Build history of the part. All positions in model axes, mm. A direction names the side the tool comes from. Give positions to 0.01 mm unless a question says otherwise; leave off trailing zeros. Loops run counter-clockwise (first coordinate to the right, second up) from the corner with the lowest first, then second, coordinate; pieces in that order, holes last. Notation, with made-up numbers: (35.25, -35.75) - (86.25, -35.75) arc R34 ccw to (86.25, -0.75) - close; hole circle Ø11 at (72, -7.75). An arc over 180 degrees is marked (long way). Return JSON: item names as keys, results as strings. Group by question number.
1) Drop flat-ended pins along their axis: pin 1 (3 mm diameter, centred on x = -4, z = 44, fed in from +Y); pin 2 (3 mm diameter, centred on x = -0.5, y = 0, fed in from +Z); pin 3 (6 mm diameter, centred on x = 3.5, z = 26, fed in from +Y). Give the stop position or say it passes through.
2) Mould opens along X. For faces 1 (the face through (0, -3, 75)), 2 (the face through (-5, 0, 37)), 3 (the face through (-0.151, 0.678, 16.986)) say: released by +X, released by -X, zero draft, split by the parting line, or undercut.
3) Drill centre lines: probe 1 along Y at (x, z) = (0, 3.5); probe 2 along Y at (x, z) = (-2, 69.5); probe 3 along Y at (x, z) = (-0.25, 28). Where is each one in solid material? Low to high. Write a range as from..to.
4) Slice it at A-A (z = 69.5). List the corners of the cut face in (x, y).
5) 3-axis set-ups, long thin cutter, end or side, ignore diameter. For faces 4 (the face through (0, 3, 75)), 5 (the face through (0, -2, 60)), 6 (the face through (0.867, 3.905, 7.605)): which of +Z, -Z, +X, -X, +Y, -Y reach the whole face in a straight line?
```python
from build123d import *

# Parameters (mm, degrees)
F0_R     = 5
F1_DEPTH = 75
F3_D     = 8
F3_DEPTH = 15
F3_TIP   = 2.4034424761
F4_W     = 2
F4_H     = 30
F5_DEPTH = 12.5


with BuildPart() as f1:
    # F0 (on Top) → F1 (new body)
    with BuildSketch(Plane.XY):
        Circle(F0_R)
    extrude(amount=F1_DEPTH)

    # F3
    with Locations(Plane(origin=(0, 0, 0), x_dir=(1, 0, 0), z_dir=(0, 0, -1))):
        with Locations((0, 0)):
            Hole(F3_D / 2, depth=F3_DEPTH)
            with Locations((0, 0, -(F3_DEPTH + F3_TIP / 2))):  # 118° drill point
                Cone(0, F3_D / 2, F3_TIP, mode=Mode.SUBTRACT)

    # F4 (on Right) → F5 (cut, symmetric)
    with BuildSketch(Plane.YZ):
        with Locations((-1, 60)):
            Rectangle(F4_W, F4_H)
        with Locations((1, 60)):
            Rectangle(F4_W, F4_H)
    extrude(amount=F5_DEPTH, both=True, mode=Mode.SUBTRACT)


solid = f1.part
```
Results:
{
 "1": {"pin 1": "y = 4.33", "pin 2": "z = 45", "pin 3": "y = 4.97"},
 "2": {"face 1": "zero draft", "face 2": "split by the parting line", "face 3": "undercut"},
 "3": {"probe 1": "-5..-4, 4..5", "probe 2": "-4.58..-2, 2..4.58", "probe 3": "-4.99..4.99"},
 "4": {"outline": "(-4.58, -2) arc R5 ccw to (4.58, -2) - close; (-4.58, 2) - (4.58, 2) arc R5 ccw to start"},
 "5": {"face 4": "+Z, +X, -X, +Y, -Y", "face 5": "+Z, +X, -X", "face 6": "-Z"}
}
